Work out the finished part from the listing and answer in its coordinate system (mm). A direction names the side the tool comes from. Round coordinates to 2 decimals unless told otherwise and drop trailing zeros. Loops run counter-clockwise (first coordinate to the right, second up) from the corner with the lowest first, then second, coordinate; pieces in that order, holes last. Notation, with made-up numbers: (-33.75, 9.25) -> (24.25, 9.25) arc R23 cw to (24.25, 42.25) -> close; hole circle Ø8 at (83.25, 12.25). An arc over 180 degrees is marked (long way). Write item = value, one per line. Start each with the question number.
```python
from build123d import *

# Parameters (mm, degrees)
F1_DEPTH = 2


with BuildPart() as f1:
    # F0 (on Top) → F1 (new body)
    with BuildSketch(Plane.XY):
        with BuildLine():
            Line((0, 1), (0, 0))
            Line((0, 0), (17.5, 0))
            Line((17.5, 0), (17.5, 3))
            Line((17.5, 3), (10, 3))
            ThreePointArc((10, 3), (9.200786, 2.891584), (8.459337, 2.574171))
            Line((8.459337, 2.574171), (6.540663, 1.425829))
            ThreePointArc((6.540663, 1.425829), (5.799214, 1.108416), (5, 1))
            Line((5, 1), (0, 1))
        make_face()
    extrude(amount=F1_DEPTH)

    # F2: F1 across face


with BuildPart() as f1_1:
    add(f1.part)
    add(f1.part.mirror(Plane(origin=(8.75, 0, 1), x_dir=(1, 0, 0), z_dir=(0, -1, 0))))

    # F3: F1 across face


with BuildPart() as f1_2:
    add(f1_1.part)
    add(f1_1.part.mirror(Plane(origin=(0, 0, 1), x_dir=(0, -1, 0), z_dir=(-1, 0, 0))))


solid = f1_2.part
```
Item 1: Section B-B (z = 1.25) is taken. Determine the outline of the cut face in (x, y), then the cut area to 3 significant figures.
Item 2: Find the intervals of material crossed by line 1 along X through (y, z) = (2.25, 1.55); line 2 along Y through (x, z) = (0, 1); line 3 along X through (y, z) = (2.5, 0.4), in increasing order. Write a range as [from, to].
Item 3: Section C-C (x = 3.5) is taken. Determine the outline of the cut face in (y, z).
Item 4: Section D-D (x = 7.5) is taken. Determine the outline of the cut face in (y, z), then the cut area to 3 significant figures.
Item 5: A tool of negligible diameter and unlimited length cuts with its end or side. For faces 5 (the flat face through (0, -1, 1)), 6 (the flat face through (0, 0, 0)), 7 (the cylindrical face through (9.212, 2.895, 0.986)), from which of +Z, -Z, +X, -X, +Y, -Y can it reach the whole face along a straight path? Write none if from no direction.
Item 6: Section A-A (y = 2) is taken. Determine the outline of the cut face in (x, z).
Item 7: The mould has two halves that part along X. Classify faces 1 (the flat face through (17.5, 0, 1)), 2 (the flat face through (-17.5, 0, 1)), 3 (the flat face through (-14, -3, 1)), 4 (the cylindrical face through (5.81, -1.11, 0.99)): pulls with the +X half, pulls with the -X half, needs draft (parallel to the pull), parting line crosses it, or undercut.
Worked answers:
q1.outline = (-17.5, -3) -> (-10, -3) arc R3 ccw to (-8.46, -2.57) -> (-6.54, -1.43) arc R3 cw to (-5, -1) -> (5, -1) arc R3 cw to (6.54, -1.43) -> (8.46, -2.57) arc R3 ccw to (10, -3) -> (17.5, -3) -> (17.5, 3) -> (10, 3) arc R3 ccw to (8.46, 2.57) -> (6.54, 1.43) arc R3 cw to (5, 1) -> (-5, 1) arc R3 cw to (-6.54, 1.43) -> (-8.46, 2.57) arc R3 ccw to (-10, 3) -> (-17.5, 3) -> close
q1.area = 150 mm2
q2.line_1 = [-17.5, -7.92], [7.92, 17.5]
q2.line_2 = [-1, 1]
q2.line_3 = [-17.5, -8.34], [8.34, 17.5]
q3.outline = (-1, 0) -> (1, 0) -> (1, 2) -> (-1, 2) -> close
q4.outline = (-2, 0) -> (2, 0) -> (2, 2) -> (-2, 2) -> close
q4.area = 8.00 mm2
q5.face_5 = +Z, -Z, -Y
q5.face_6 = -Z, +X, -X, +Y, -Y
q5.face_7 = +Z, -Z, +Y
q6.outline = (-17.5, 0) -> (-7.5, 0) -> (-7.5, 2) -> (-17.5, 2) -> close; (7.5, 0) -> (17.5, 0) -> (17.5, 2) -> (7.5, 2) -> close
q7.face_1 = pulls with the +X half
q7.face_2 = pulls with the -X half
q7.face_3 = needs draft
q7.face_4 = undercut
